Autodesk Inventor part; units mm, degrees
ref_plane "XZ Plane" through (0, 0, 0) normal (0, 1, 0) x (-1, 0, 0)
ref_plane "XY Plane" through (0, 0, 0) normal (0, 0, 1) x (1, 0, 0)
sketch "Sketch1" plane through (0, 0, 0) normal (0, 0, 1) x (1, 0, 0)
  line L0 (0, 0) -> (203.2, 0)
  line L1 (203.2, 0) -> (203.2, 609.6)
  line L2 (203.2, 609.6) -> (0, 609.6)
  line L3 (0, 0) -> (0, 609.6) construction
  line L4 (0, 0) -> (-203.2, 0)
  line L5 (-203.2, 0) -> (-203.2, 609.6)
  line L6 (-203.2, 609.6) -> (0, 609.6)
  line L7 (-177.8, 25.4) -> (177.8, 25.4)
  line L8 (177.8, 25.4) -> (177.8, 584.2)
  line L9 (177.8, 584.2) -> (-177.8, 584.2)
  line L10 (-177.8, 584.2) -> (-177.8, 25.4)
  dimension "d1" = 609.6
  dimension "d2" = 406.4
  dimension "d3" = 25.4
  dimension "d4" = 25.4
  dimension "d5" = 25.4
  dimension "d6" = 25.4
extrude "Extrusion1" add sketch "Sketch1" along normal mid plane 25.4
properties part number "primativeBaseForShortRobot"
Geometry check sheet. Reference: the model listing, model coordinates, mm. A direction names the side the tool comes from. Coordinates: 2 decimals unless noted, no trailing zeros. Order: outer loops, then holes, each group sorted by start corner. A loop starts at its lowest first (then second) coordinate and runs counter-clockwise, first axis right, second up. Notation, with made-up numbers: (-28.5, -7) - (29.5, -7) arc R8 ccw to (29.5, 7) - close; hole circle Ø4 at (-22, 48.25). An arc over 180 degrees is marked (long way). One line per item, written item: value.
(1) Sectioned sample at C-C (z = 2). Enter the section's corners in (x, y).
Data:
outline: (-203.2, 0) - (203.2, 0) - (203.2, 609.6) - (-203.2, 609.6) - close; hole (-177.8, 25.4) - (177.8, 25.4) - (177.8, 584.2) - (-177.8, 584.2) - close
(2) Thickness scan on probe 1 along Y at (x, z) = (86, -1.5); probe 2 along X at (y, z) = (334.5, 9.75). Record the ranges inside material, lowest first. Write a range as from..to.
Data:
probe 1: y = 0..25.4, 584.2..609.6
probe 2: x = -203.2..-177.8, 177.8..203.2
(3) Sectioned sample at A-A (y = 166.5). Enter the section's corners in (x, z).
Data:
outline: (-203.2, -12.7) - (-177.8, -12.7) - (-177.8, 12.7) - (-203.2, 12.7) - close; (177.8, -12.7) - (203.2, -12.7) - (203.2, 12.7) - (177.8, 12.7) - close
(4) Access from +Z, -Z, +X, -X, +Y, -Y to the whole of each face (thin tool, end or side, straight path). Record for faces 1 (the face through (2, 584.2, 0)), 2 (the face through (203.2, 301, 0)).
Data:
face 1: +Z, -Z
face 2: +Z, -Z, +X, +Y, -Y
(5) Release check for a two-part mould opening along Y. For faces 3 (the face through (-203.2, 301, 0)), 4 (the face through (-3, 609.6, 0)), 5 (the face through (-2, 25.4, 0)), 6 (the face through (3, 0, 0)) record: +Y half, -Y half, draft (parallel to the pull), parting line (faces both ways), or undercut.
Data:
face 3: draft
face 4: +Y half
face 5: undercut
face 6: -Y half
(6) Sectioned sample at B-B (x = 149). Enter the section's corners in (y, z), and give its area (3 significant figures).
Data:
outline: (0, -12.7) - (25.4, -12.7) - (25.4, 12.7) - (0, 12.7) - close; (584.2, -12.7) - (609.6, -12.7) - (609.6, 12.7) - (584.2, 12.7) - close
area: 1,290 mm^2
